Source: CAD feature listing. Evaluate the final solid. Frame: model axes, mm. Face numbers are marked on the shaded views. A direction names the side the tool comes from. Give positions to 0.01 mm unless a question says otherwise; leave off trailing zeros. Order: outer loops, then holes, each group sorted by start corner. A loop starts at its lowest first (then second) coordinate and runs counter-clockwise, first axis right, second up. Notation, with made-up numbers: M 63,17.5 L 97,17.5 A22 cw 97,48.5 Z; hole C 19.5,40.25 d5. An arc over 180 degrees is marked long. Answer in a Markdown table with one row per item. Add a question column.
(1) Mould query, pull axis X, two halves, no side actions, for the marked faces 4, 5 and 6. Classes: pulls with the +X half, pulls with the -X half, needs draft (parallel to the pull), parting line crosses it, or undercut.
(2) Section query A-A, the plane y = 4. Return loops of the section in (x, z), plus the area to 3 significant figures.
(3) Set-up query: the marked faces 1, 2 and 3. Return all of +Z, -Z, +X, -X, +Y, -Y with unobstructed straight access to the full face (end or side cutting, diameter ignored); none if empty.
(4) Pin query (flat end, axial travel): P1, Ø3, axis at x = 0, y = -4, coming from the -Z side. Return the tip coordinate at first contact, or that it passes through.
(5) Section query B-B, the plane x = 4. Return loops of the section in (y, z), plus the area to 3 significant figures.
(6) Material intervals for line 1 along Y through (x, z) = (8, 0.85); line 2 along X through (y, z) = (4, 1.25); line 3 along Y through (x, z) = (-1.25, 0.5), sorted ascending.
from build123d import *

# Parameters (mm, degrees)
F1_DEPTH = 8
F3_W     = 8
F3_H     = 8
F3_R     = 2.4
F4_DEPTH = 1.7
F5_R     = 2.4
F6_DEPTH = 1.7


with BuildPart() as f1:
    # F0 (on Front) → F1 (new body)
    with BuildSketch(Plane.XZ):
        Polygon((-2.4, 9.6), (-4, 9.6), (-4, 0), (4, 0), (4, 9.6), (2.4, 9.6), (2.4, 11.3), (-2.4, 11.3), align=None)
    extrude(amount=F1_DEPTH)

    # F3 (on plane+point) → F4 (cut, through all)
    with BuildSketch(Plane.XY.offset(11.3)):
        with Locations((0, -4)):
            Rectangle(F3_W, F3_H)
        with Locations((0, -4)):
            Circle(F3_R, mode=Mode.SUBTRACT)
    extrude(amount=-F4_DEPTH, mode=Mode.SUBTRACT)

    # F5 (on Top) → F6 (cut)
    with BuildSketch(Plane.XY):
        with Locations((0, -4)):
            Circle(F5_R)
    extrude(amount=F6_DEPTH, mode=Mode.SUBTRACT)

    # F8: F1 across plane


with BuildPart() as f1_1:
    add(f1.part)
    add(f1.part.mirror(Plane.YZ.offset(4)))

    # F9: F1 across plane


with BuildPart() as f1_2:
    add(f1_1.part)
    add(f1_1.part.mirror(Plane.XZ))


solid = f1_2.part
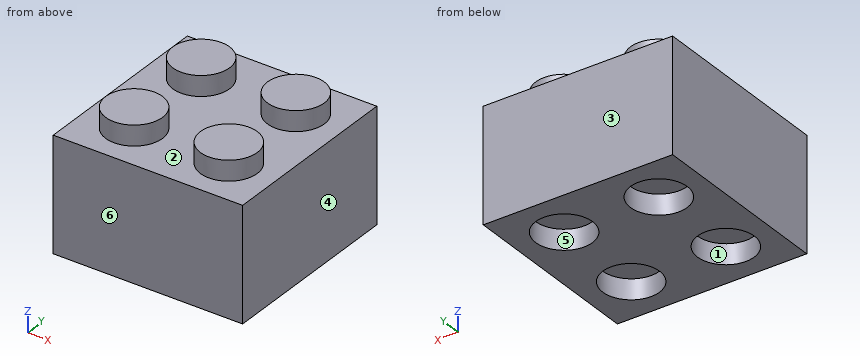
Values follow:
| question | item | result |
|---|---|---|
| 1 | face 4 | pulls with the +X half |
| 1 | face 5 | undercut |
| 1 | face 6 | needs draft |
| 2 | outline | M -4,0 L -2.4,0 L -2.4,1.7 L 2.4,1.7 L 2.4,0 L 5.6,0 L 5.6,1.7 L 10.4,1.7 L 10.4,0 L 12,0 L 12,9.6 L 10.4,9.6 L 10.4,11.3 L 5.6,11.3 L 5.6,9.6 L 2.4,9.6 L 2.4,11.3 L -2.4,11.3 L -2.4,9.6 L -4,9.6 Z |
| 2 | area | 154 mm² |
| 3 | face 1 | -Z |
| 3 | face 2 | +Z |
| 3 | face 3 | +Z, -Z, +X, -X, +Y |
| 4 | P1 | stops at z = 1.7 |
| 5 | outline | M -8,0 L 8,0 L 8,9.6 L -8,9.6 Z |
| 5 | area | 154 mm² |
| 6 | line 1 | y = -8 to -6.4, -1.6 to 1.6, 6.4 to 8 |
| 6 | line 2 | x = -4 to -2.4, 2.4 to 5.6, 10.4 to 12 |
| 6 | line 3 | y = -8 to -6.05, -1.95 to 1.95, 6.05 to 8 |
